Geometry: final body of the model. Coordinates: model frame, mm. A direction names the side the tool comes from. Give positions to 0.01 mm unless a question says otherwise; leave off trailing zeros. Write each loop counter-clockwise with the first axis right and the second up, starting at its lowest first coordinate (ties: lowest second). Pieces come first, ordered by that corner, then holes.
Q1. Cut plane D-D on y = 3.75. Return the cut outline in (x, z) (3 decimals), plus the area to 3 significant figures.
Q2. Reachability of faces 1 (the face through (19, 19.05, 21)), 2 (the face through (0, 15, 6)), 3 (the face through (24.5, 5.2, 13.6)), 4 (the face through (19, 6.35, 3)), 5 (the face through (8, 12, 12)) from +Z, -Z, +X, -X, +Y, -Y: full face, straight path, thin tool, end or side. Return the list, or none.
Q3. Line query: L1, parallel to Y at x = 17.5, z = 22; L2, parallel to Y at x = 23, z = 4; L3, parallel to Z at x = 31, y = 6.75. Output: solid intervals per line, ascending.
Q4. Draft query along X for faces 6 (the face through (19, 0, 7)), 7 (the face through (19, 3, 6.35)), 8 (the face through (4.8, 21.8, 17.5)), 9 (the face through (38.1, 15, 6)). Return one class per face: pulls with the +X half, pulls with the -X half, needs draft (parallel to the pull), parting line crosses it, or undercut.
Q5. Cut plane A-A on x = 14.5. Return the cut outline in (y, z).
Q6. Pin query (flat end, axial travel): pin 1 (12 mm diameter, centred on x = 34, y = 10.5, fed in from -Z); pin 2 (2 mm diameter, centred on x = 11.5, y = 5.5, fed in from +Z); pin 3 (3 mm diameter, centred on x = 24.5, z = 22.5, fed in from -Y); pin 4 (3 mm diameter, centred on x = 21.5, y = 4, fed in from -Z). Return the tip coordinate at first contact, or that it passes through.
Q7. Cut plane C-C on z = 4. Return the cut outline in (x, y) (3 decimals).
Q8. Cut plane B-B on y = 14.25. Return the cut outline in (x, z).
```python
from build123d import *

# Parameters (mm, degrees)
F0_W      = 12.7
F0_H      = 6.35
F1_DEPTH  = 25.4
F3_DEPTH  = 6.351
F4_DEPTH  = 19.05
F6_DEPTH  = 19.05
F7_DEPTH  = 25.4
F9_DEPTH  = 38.101
F10_DEPTH = 25.4
F12_DEPTH = 25.401


with BuildPart() as f1:
    # F0 (on Top) → F1 (new body)
    with BuildSketch(Plane.XY):
        Polygon((25.4, 25.4), (12.7, 25.4), (12.7, 19.05), (19.05, 19.05), (25.4, 19.05), align=None)
        with Locations((6.35, 22.225)):
            Rectangle(F0_W, F0_H)
        with Locations((31.75, 22.225)):
            Rectangle(F0_W, F0_H)
    extrude(amount=F1_DEPTH)

    # F2 (on face) → F3 (cut, through all)
    with BuildSketch(Plane.XZ.offset(-19.05)):
        Polygon((12.7, 25.4), (0, 25.4), (0, 12.7), align=None)
        Polygon((38.1, 25.4), (25.4, 25.4), (38.1, 12.7), align=None)
    extrude(amount=-F3_DEPTH, mode=Mode.SUBTRACT)



with BuildPart() as f4:
    # F0 (on Top) → F4 (new body)
    with BuildSketch(Plane.XY):
        Polygon((19.05, 19.05), (0, 0), (9.525, 0), (9.525, 6.35), (28.575, 6.35), (28.575, 0), (38.1, 0), align=None)
    extrude(amount=F4_DEPTH)

    # F5 (on face) → F6 (cut)
    with BuildSketch(Plane.XZ):
        Polygon((38.1, 19.05), (28.575, 19.05), (28.575, 9.525), (38.1, 0), align=None)
        Polygon((0, 19.05), (0, 0), (19.05, 19.05), align=None)
    extrude(amount=-F6_DEPTH, mode=Mode.SUBTRACT)


with BuildPart() as f1_1:
    add(f1.part)

    add(f4.part)  # F7 merges F4
    # F0 (on Top) → F7 (join)
    with BuildSketch(Plane.XY):
        Polygon((38.1, 19.05), (25.4, 19.05), (19.05, 19.05), (38.1, 0), align=None)
        Polygon((12.7, 19.05), (0, 19.05), (0, 0), (19.05, 19.05), align=None)
    extrude(amount=F7_DEPTH)

    # F8 (on face) → F9 (cut, through all)
    with BuildSketch(Plane.YZ.offset(38.1)):
        Polygon((0, 0), (19.05, 19.05), (19.05, 25.4), (0, 25.4), align=None)
    extrude(amount=-F9_DEPTH, mode=Mode.SUBTRACT)

    # F5 (on face) → F10 (join)
    with BuildSketch(Plane.XZ):
        Polygon((19.05, 19.05), (0, 0), (9.525, 0), (9.525, 6.35), (28.575, 6.35), (28.575, 9.525), align=None)
        Polygon((28.575, 6.35), (28.575, 0), (38.1, 0), (28.575, 9.525), align=None)
    extrude(amount=-F10_DEPTH)

    # F11 (on face) → F12 (cut, through all)
    with BuildSketch(Plane.XZ):
        Polygon((6.35, 19.05), (0, 19.05), (0, 12.7), align=None)
        Polygon((38.1, 12.7), (38.1, 19.05), (31.75, 19.05), align=None)
    extrude(amount=-F12_DEPTH, mode=Mode.SUBTRACT)


solid = f1_1.part
```
Data:
1. outline: (0, 0) - (9.525, 0) - (9.525, 6.35) - (28.575, 6.35) - (28.575, 0) - (38.1, 0) - (38.1, 3.75) - (34.35, 3.75) - (19.05, 19.05) - (3.75, 3.75) - (0, 3.75) - close
1. area: 256 mm2
2. face 1: +Z, +X, -X, -Y
2. face 2: +Z, -Z, -X, +Y, -Y
2. face 3: +Z, +X, -Y
2. face 4: -Z, -Y
2. face 5: +Z, -X, -Y
3. L1: y = 19.05 to 25.4
3. L2: y = 6.35 to 25.4
3. L3: z = 0 to 7.1
4. face 6: needs draft
4. face 7: undercut
4. face 8: pulls with the -X half
4. face 9: pulls with the +X half
5. outline: (0, 6.35) - (6.35, 6.35) - (6.35, 0) - (25.4, 0) - (25.4, 25.4) - (19.05, 25.4) - (19.05, 19.05) - (14.5, 14.5) - (0, 14.5) - close
6. pin 1: stops at z = 0
6. pin 2: stops at z = 12.5
6. pin 3: stops at y = 19.05
6. pin 4: stops at z = 6.35
7. outline: (0, 4) - (4, 4) - (4, 0) - (9.525, 0) - (9.525, 6.35) - (28.575, 6.35) - (28.575, 0) - (34.1, 0) - (34.1, 4) - (38.1, 4) - (38.1, 25.4) - (0, 25.4) - close
8. outline: (0, 0) - (38.1, 0) - (38.1, 12.7) - (36.55, 14.25) - (23.85, 14.25) - (19.05, 19.05) - (14.25, 14.25) - (1.55, 14.25) - (0, 12.7) - close
